Build history of the part. All positions in model axes, mm. Face numbers are marked on the shaded views. A direction names the side the tool comes from. Give positions to 0.01 mm unless a question says otherwise; leave off trailing zeros. Order: outer loops, then holes, each group sorted by start corner. A loop starts at its lowest first (then second) coordinate and runs counter-clockwise, first axis right, second up. Notation, with made-up numbers: M 38.25,-5.75 L 71.25,-5.75 A14 ccw 71.25,10.25 Z; hole C -12,7.25 d2. An arc over 180 degrees is marked long. One line per item, written item: value.
from build123d import *

# Parameters (mm, degrees)
SKETCH_1_W               = 5.4
SKETCH_1_H               = 65
EXTRUDE_1_DEPTH          = 2.7
CUT_EXTRUDE_1_DEPTH      = 33.723538928
CUT_EXTRUDE_1_DEPTH_BACK = 33.723538928
EXTRUDE_2_DEPTH          = 40
CHAMFER_1_SIZE           = 5
CUT_EXTRUDE_2_DEPTH      = 73.576392116
CUT_EXTRUDE_2_DEPTH_BACK = 73.576392116
SKETCH_6_R               = 1.35


with BuildPart() as part:
    # 草图1 → 凸台-拉伸1 (new, symmetric)
    with BuildSketch(Plane(origin=(0, 0, 0), x_dir=(1, 0, 0), z_dir=(0, 1, 0))):
        Rectangle(SKETCH_1_W, SKETCH_1_H)
    extrude(amount=EXTRUDE_1_DEPTH, both=True)

    # 草图3 → 切除-拉伸1 (cut, two sides: drawn at the far end of the back side and taken through both)
    with BuildSketch(Plane(origin=(0, 0, 0), x_dir=(0, 0, -1), z_dir=(1, 0, 0)).offset(-CUT_EXTRUDE_1_DEPTH_BACK)):
        Polygon((29.07653718, 2.7), (32.5, 0.72346282), (32.5, 2.7), align=None)
        Polygon((32.5, -2.7), (32.5, 0.72346282), (30.52346282, -2.7), align=None)
    extrude(amount=CUT_EXTRUDE_1_DEPTH + CUT_EXTRUDE_1_DEPTH_BACK, mode=Mode.SUBTRACT)

    # 草图4 → 凸台-拉伸2 (add, symmetric)
    with BuildSketch(Plane(origin=(0, 0, 0), x_dir=(0, 0, -1), z_dir=(1, 0, 0))):
        with BuildLine():
            ThreePointArc((-29.382308546, 2.7), (-33.641154273, 1.558845727), (-32.5, -2.7))
            Line((-32.5, -2.7), (-29.382308546, 2.7))
        make_face()
    extrude(amount=EXTRUDE_2_DEPTH, both=True)

    # 倒角1
    chamfer_1_edges = [part.edges().sort_by_distance(p)[0] for p in [
        (-2.7, 0, 30.941154273),
        (2.7, 0, 30.941154273),
    ]]
    chamfer(chamfer_1_edges, length=CHAMFER_1_SIZE)

    # 草图6 → 切除-拉伸2 (cut, two sides: drawn at the far end of the back side and taken through both)
    with BuildSketch(Plane(origin=(0, -13.892047107, -24.06173141), x_dir=(-1, 0, 0), z_dir=(0, -0.4999999999999933, -0.8660254037844425)).offset(-CUT_EXTRUDE_2_DEPTH_BACK)):
        with Locations(Location((0, 14.17653718, 0), (0, 0, 90))):
            Circle(SKETCH_6_R)
    extrude(amount=CUT_EXTRUDE_2_DEPTH + CUT_EXTRUDE_2_DEPTH_BACK, mode=Mode.SUBTRACT)


solid = part.part
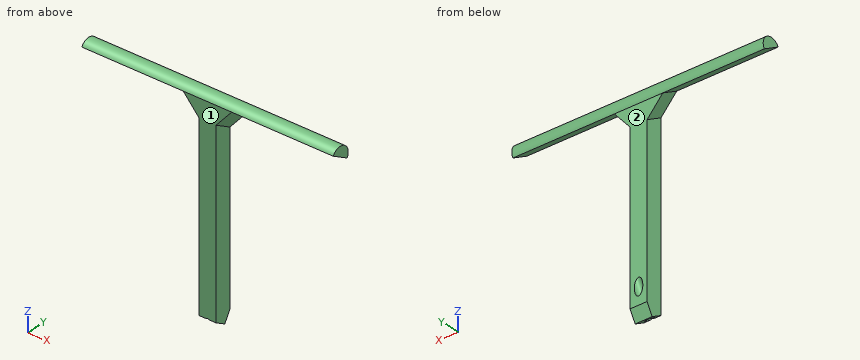
1) Tool access for the marked faces 1 and 2: list every direction of +Z, -Z, +X, -X, +Y, -Y with a clear straight run to the whole face (end or side of a thin tool).
Check values:
face 1: +Z, -Z, +X, -X, -Y
face 2: -Z, +X, -X, +Y
2) Pin check, flat tips, straight feed: pin 1 (1 mm diameter, centred on y = 2.5, z = 2.5, fed in from -X); pin 2 (17 mm diameter, centred on x = -2.5, z = -8, fed in from +Y); pin 3 (1 mm diameter, centred on y = 2, z = 23.5, fed in from -X). Stop position of each tip, or through.
Check values:
pin 1: x = -2.7
pin 2: y = 2.7
pin 3: x = -2.76
3) Saw through at B-B, the plane z = 4.5. Write the cut outline in (x, y).
Check values:
outline: M -2.7,-2.7 L 2.7,-2.7 L 2.7,2.7 L -2.7,2.7 Z
4) Drill centre lines: probe 1 along Y at (x, z) = (-2.5, 27.5); probe 2 along Z at (x, y) = (-3, 0.9). Where is each one in solid material? Low to high. Write a range as from..to.
Check values:
probe 1: -2.7..2.7
probe 2: 24.99..33.93
